from build123d import *

# Parameters (mm, degrees)
SKETCH1_W           = 60
SKETCH1_H           = 40
BOSS_EXTRUDE1_DEPTH = 24.5
SKETCH2_R           = 15
SKETCH2_R_2         = 14
BOSS_EXTRUDE2_DEPTH = 1
SKETCH3_R           = 3.175
SKETCH3_R_2         = 1.5
CUT_EXTRUDE1_DEPTH  = 10
SKETCH4_R           = 3.175
SKETCH4_R_2         = 1.5
CUT_EXTRUDE2_DEPTH  = 10
SKETCH5_R           = 1
SKETCH5_W           = 12
SKETCH5_H           = 4
CUT_EXTRUDE3_DEPTH  = 5
SKETCH6_R           = 2.5
SKETCH6_R_2         = 2
BOSS_EXTRUDE4_DEPTH = 5


with BuildPart() as part:
    # Sketch1 → Boss-Extrude1 (new body)
    with BuildSketch(Plane.XY):
        with Locations((30, 20)):
            Rectangle(SKETCH1_W, SKETCH1_H)
    extrude(amount=BOSS_EXTRUDE1_DEPTH)

    # Sketch2 → Boss-Extrude2 (add)
    with BuildSketch(Plane(origin=(0, 0, 0), x_dir=(-1, 0, 0), z_dir=(0, 0, -1))):
        with Locations((-30, 20)):
            Circle(SKETCH2_R)
        with Locations((-30, 20)):
            Circle(SKETCH2_R_2, mode=Mode.SUBTRACT)
    extrude(amount=BOSS_EXTRUDE2_DEPTH)

    # Sketch3 → Cut-Extrude1 (cut)
    with BuildSketch(Plane.ZY):
        with Locations((4.5, 20)):
            Circle(SKETCH3_R)
        with Locations((4.5, 28)):
            Circle(SKETCH3_R_2)
        with Locations((4.5, 12)):
            Circle(SKETCH3_R_2)
    cut_extrude1 = extrude(amount=-CUT_EXTRUDE1_DEPTH, mode=Mode.SUBTRACT)

    # Mirror1: Cut-Extrude1 across plane
    add(cut_extrude1.mirror(Plane(origin=(30, 0, 0), x_dir=(0, 0, 1), z_dir=(1, 0, 0))), mode=Mode.SUBTRACT)

    # Sketch4 → Cut-Extrude2 (cut)
    with BuildSketch(Plane(origin=(0, 40, 0), x_dir=(1, 0, 0), z_dir=(0, 1, 0))):
        with Locations((30, -4.5)):
            Circle(SKETCH4_R)
        with Locations((38, -4.5)):
            Circle(SKETCH4_R_2)
        with Locations((22, -4.5)):
            Circle(SKETCH4_R_2)
    cut_extrude2 = extrude(amount=-CUT_EXTRUDE2_DEPTH, mode=Mode.SUBTRACT)

    # Mirror2: Cut-Extrude2 across plane
    add(cut_extrude2.mirror(Plane(origin=(0, 20, 0), x_dir=(0, 0, 1), z_dir=(0, -1, 0))), mode=Mode.SUBTRACT)

    # Sketch5 → Cut-Extrude3 (cut)
    with BuildSketch(Plane.XY.offset(24.5)):
        with Locations((21, 6)):
            Circle(SKETCH5_R)
        with Locations((39, 6)):
            Circle(SKETCH5_R)
        with Locations((30, 6)):
            Rectangle(SKETCH5_W, SKETCH5_H)
    extrude(amount=-CUT_EXTRUDE3_DEPTH, mode=Mode.SUBTRACT)

    # Sketch6 → Boss-Extrude4 (add)
    with BuildSketch(Plane.XY.offset(24.5)):
        with Locations((51.35, 12)):
            Circle(SKETCH6_R)
        with Locations((51.35, 12)):
            Circle(SKETCH6_R_2, mode=Mode.SUBTRACT)
        with Locations((51.35, 28)):
            Circle(SKETCH6_R)
        with Locations((51.35, 28)):
            Circle(SKETCH6_R_2, mode=Mode.SUBTRACT)
    extrude(amount=BOSS_EXTRUDE4_DEPTH)


solid = part.part
Could you check a few things on this model? Use its own coordinates, in mm. A direction names the side the tool comes from. Round coordinates to 2 decimals unless told otherwise and drop trailing zeros. Order: outer loops, then holes, each group sorted by start corner. A loop starts at its lowest first (then second) coordinate and runs counter-clockwise, first axis right, second up.
(1) Please list where these lines run through material, in increasing order: line 1 along X through (y, z) = (3, 4.5) (3 decimals); line 2 along Y through (x, z) = (56.75, 4.5) (3 decimals); line 3 along Y through (x, z) = (39, 22).
Response values:
line 1: x = 0 to 20.5, 23.5 to 26.825, 33.175 to 36.5, 39.5 to 60
line 2: y = 0 to 10.5, 13.5 to 16.825, 23.175 to 26.5, 29.5 to 40
line 3: y = 0 to 5, 7 to 40
(2) Imagine slicing it at D-D (z = 27). Write out the boundary of the cut face in (x, y), plus the area to 3 significant figures.
Response values:
outline: circle Ø5 at (51.35, 12); circle Ø5 at (51.35, 28); hole circle Ø4 at (51.35, 12); hole circle Ø4 at (51.35, 28)
area: 14.1 mm2
(3) Imagine slicing it at B-B (z = 21.5). Write out the boundary of the cut face in (x, y).
Response values:
outline: (0, 0) - (60, 0) - (60, 40) - (0, 40) - close; hole circle Ø2 at (21, 6); hole (24, 4) - (36, 4) - (36, 8) - (24, 8) - close; hole circle Ø2 at (39, 6)
(4) Imagine slicing it at C-C (y = 20). Write out the boundary of the cut face in (x, z) (3 decimals).
Response values:
outline: (0, 0) - (15, 0) - (15, -1) - (16, -1) - (16, 0) - (44, 0) - (44, -1) - (45, -1) - (45, 0) - (60, 0) - (60, 1.325) - (50, 1.325) - (50, 7.675) - (60, 7.675) - (60, 24.5) - (0, 24.5) - (0, 7.675) - (10, 7.675) - (10, 1.325) - (0, 1.325) - close
(5) Which directions (+Z, -Z, +X, -X, +Y, -Y) give clear straight access to the entire face, cutting with the end or side of a thin tool? Please do faces 1 (the flat face through (30, 8, 22)), 2 (the cylindrical face through (36.8, 35.1, 5.4)), 3 (the flat face through (30, 20, 0)), 4 (the flat face through (10, 20, 4)).
Response values:
face 1: +Z
face 2: +Y
face 3: -Z
face 4: -X
(6) Imagine slicing it at A-A (x = 55). Write out the boundary of the cut face in (y, z) (3 decimals), plus the area to 3 significant figures.
Response values:
outline: (0, 0) - (40, 0) - (40, 24.5) - (0, 24.5) - close; hole circle Ø3 at (12, 4.5); hole circle Ø6.35 at (20, 4.5); hole circle Ø3 at (28, 4.5)
area: 934 mm2
(7) If we mould it in two halves opening along Y, with no side actions, what happens to faces 5 (the flat face through (22, 10, 4)), 6 (the cylindrical face through (20.5, 4.93, 4.43)), 7 (the flat face through (22, 30, 4)), 8 (the flat face through (39, 6, 19.5))? For each: released by +Y, released by -Y, zero draft, split by the parting line, or undercut.
Response values:
face 5: released by -Y
face 6: zero draft
face 7: released by +Y
face 8: undercut
(8) I'm going to push flat-ended pins straight in: pin 1 (4 mm diameter, centred on x = 17.5, y = 18, fed in from +Z); pin 2 (0.9 mm diameter, centred on x = 38.5, z = 5, fed in from -Y); pin 3 (4 mm diameter, centred on y = 20, z = 4.5, fed in from +X). Where does each tip first touch, or does it pass through?
Response values:
pin 1: stops at z = 24.5
pin 2: stops at y = 10
pin 3: stops at x = 50
